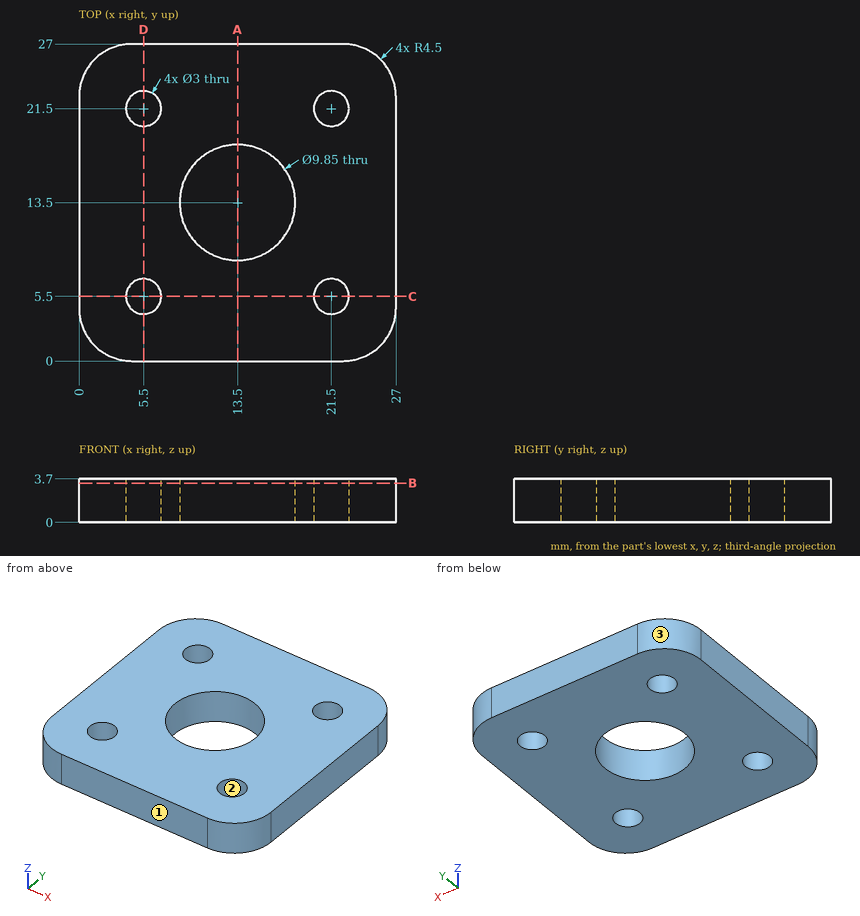
Design review of the part shown in the three views and the two pictorial views. Dimensions are in mm from the part's minimum x, y and z. Give positions to 0.01 mm unless a question says otherwise; leave off trailing zeros. Write each loop counter-clockwise with the first axis right and the second up, starting at its lowest first coordinate (ties: lowest second). Pieces come first, ordered by that corner, then holes. Notation, with made-up numbers: M 22,68 L 47,68 A13 ccw 47,74 Z; hole C 1.5,4.5 d5. An arc over 180 degrees is marked long. One line per item, written item: value.
1) Take a section at B-B, the plane z = 3.35. Write out the cut boundary in (x, y) (3 decimals), then the cut area to 3 significant figures.
Results are:
outline: M 0,4.5 A4.5 ccw 4.5,0 L 22.5,0 A4.5 ccw 27,4.5 L 27,22.5 A4.5 ccw 22.5,27 L 4.5,27 A4.5 ccw 0,22.5 Z; hole C 5.5,5.5 d3; hole C 5.5,21.5 d3; hole C 13.5,13.5 d9.85; hole C 21.5,5.5 d3; hole C 21.5,21.5 d3
area: 607 mm²
2) For line 1 (Y direction, x = 21.5, z = 2.15); line 2 (X direction, y = 13.25, z = 3.5); line 3 (Y direction, x = 4.5, z = 1.1), list the stretches that pass through material, from the lowest coordinate up. Write a range as from..to.
Results are:
line 1: y = 0..4, 7..20, 23..27
line 2: x = 0..8.58, 18.42..27
line 3: y = 0..4.38, 6.62..20.38, 22.62..27
3) Take a section at A-A, the plane x = 13.5. Write out the cut boundary in (y, z) (3 decimals), then the cut area to 3 significant figures.
Results are:
outline: M 0,0 L 8.575,0 L 8.575,3.7 L 0,3.7 Z; M 18.425,0 L 27,0 L 27,3.7 L 18.425,3.7 Z
area: 63.5 mm²
4) The part is to be moulded in two halves that separate along X. For the marked faces 1, 2 and 3, say which applies: +X half, -X half, draft (parallel to the pull), parting line (faces both ways), or undercut.
Results are:
face 1: draft
face 2: undercut
face 3: -X half
5) For P1, Ø1.5, axis at y = 23.5, z = 3, coming from the -X side; P2, Ø1, axis at x = 24, z = 3, coming from the -Y side, all flat-tipped, find the tip position at first contact; note any pin that passes through.
Results are:
P1: stops at x = 0.01
P2: stops at y = 0.11
6) Take a section at C-C, the plane y = 5.5. Write out the cut boundary in (x, z), then the cut area to 3 significant figures.
Results are:
outline: M 0,0 L 4,0 L 4,3.7 L 0,3.7 Z; M 7,0 L 20,0 L 20,3.7 L 7,3.7 Z; M 23,0 L 27,0 L 27,3.7 L 23,3.7 Z
area: 77.7 mm²
